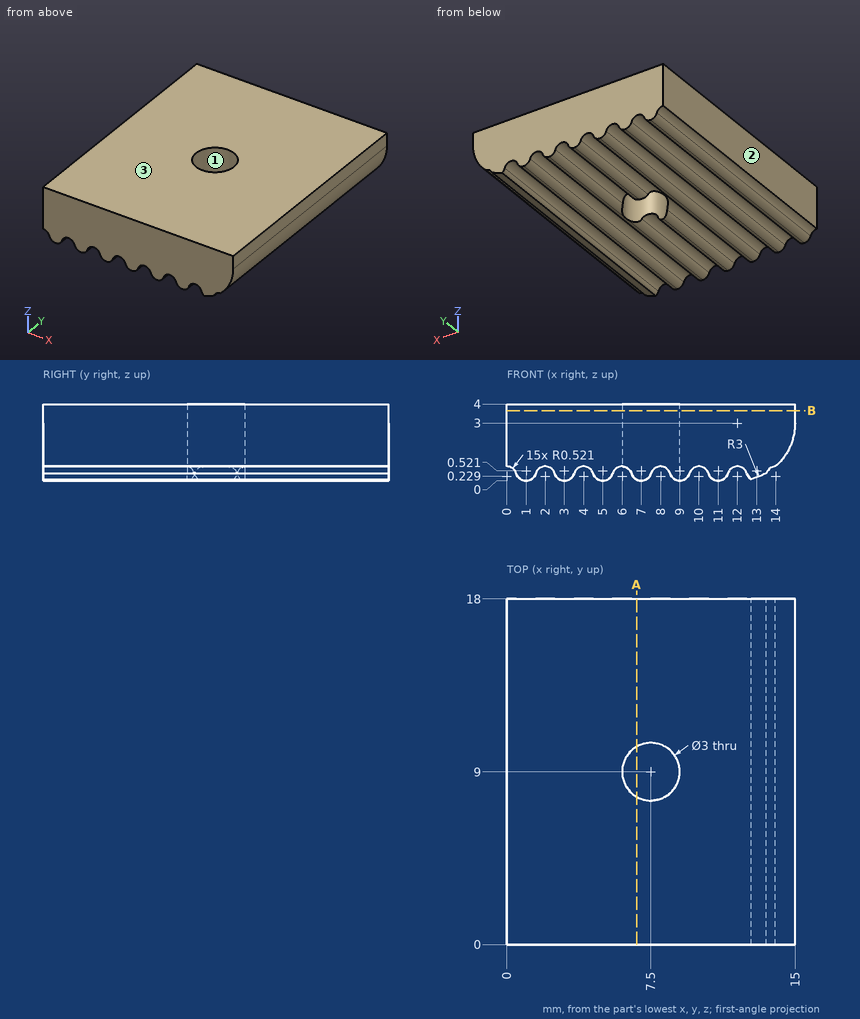
Answer from the drawing. Dimensions are ordinates in mm from the lowest x, y and z of the part. Round coordinates to 2 decimals unless told otherwise and drop trailing zeros. Write each loop counter-clockwise with the first axis right and the second up, starting at its lowest first coordinate (ties: lowest second). Pieces come first, ordered by that corner, then holes. Notation, with made-up numbers: M -3,15 L 36,15 A28 ccw 36,42 Z; hole C 13,45.5 d10. An arc over 180 degrees is marked long. Write each question's results on one line, items separated by ' | '. Start each with the question number.
Item 1: Find section B-B on z = 3.65. Write down the section's boundary in (x, y), and give its area (3 significant figures).
Item 2: Given pin 1 Ø1.5 at (y, z) = (9, 2) entering from +X, flat-ended and moving along its own axis, determine where the tip first touches the part or whether it passes through.
Item 3: Straight lines are drawn through the part: probe 1 along Y at (x, z) = (7.5, 3.1); probe 2 along Y at (x, z) = (6.5, 2.25); probe 3 along X at (y, z) = (9.5, 1) (1 decimal). For each, find the intervals that lie inside material, in ascending order.
Item 4: The mould has two halves that part along X. Classify the marked faces 1, 2 and 3: +X half, -X half, draft (parallel to the pull), parting line (faces both ways), or undercut.
Item 5: Find section A-A on x = 6.75. Write down the section's boundary in (y, z), and give its area (3 significant figures).
Answer block:
1) outline: M 0,0 L 15,0 L 15,18 L 0,18 Z; hole C 7.5,9 d3 | area: 263 mm²
2) pin 1: stops at x = 14.99
3) probe 1: y = 0 to 7.5, 10.5 to 18 | probe 2: y = 0 to 7.88, 10.12 to 18 | probe 3: x = 0 to 6.1, 8.9 to 14.2
4) face 1: undercut | face 2: -X half | face 3: draft
5) outline: M 0,0.06 L 7.7,0.06 L 7.7,4 L 0,4 Z; M 10.3,0.06 L 18,0.06 L 18,4 L 10.3,4 Z | area: 60.6 mm²
